Could you check a few things on this model? Use its own coordinates, in mm. A direction names the side the tool comes from. Give positions to 0.01 mm unless a question says otherwise; leave off trailing zeros. Order: outer loops, then holes, each group sorted by start corner. A loop starts at its lowest first (then second) coordinate and runs counter-clockwise, first axis right, second up. Notation, with made-up numbers: (-16, -6) - (34, -6) arc R19 cw to (34, 1) - close; hole circle Ø7 at (88.5, 12). An arc over 180 degrees is marked (long way). Put each result on its own line as item: value.
from build123d import *

# Parameters (mm, degrees)
EXTRUDE_THIN1_DEPTH             = 38.1
BOSS_EXTRUDE1_DEPTH             = 3.175
F_8_CLEARANCE_HOLE1_D           = 4.9149
FILLET1_R                       = 3.175
F_1_2_0_5_DIAMETER_HOLE1_D      = 12.7
F_9_64_0_14063_DIAMETER_HOLE1_D = 3.572002


with BuildPart() as part:
    # Sketch1 → Extrude-Thin1 (new body)
    with BuildSketch(Plane.XY):
        Polygon((-450.568590055, 3232.318777264), (-413.513639003, 3223.079940323), (-431.947583815, 3149.145425944), (-469.0030385, 3158.382242922), (-468.235104419, 3161.462973719), (-434.260212597, 3152.994048962), (-417.362429953, 3220.76735341), (-451.336692074, 3229.238088333), align=None)
    extrude(amount=-EXTRUDE_THIN1_DEPTH)

    # Sketch2 → Boss-Extrude1 (add)
    with BuildSketch(Plane(origin=(0, 0, -38.1), x_dir=(-1, 0, 0), z_dir=(0, 0, -1))):
        Polygon((413.513639003, 3223.079940323), (431.947583815, 3149.145425944), (469.0030385, 3158.382242922), (450.568590055, 3232.318777264), align=None)
    extrude(amount=-BOSS_EXTRUDE1_DEPTH)

    # #8 Clearance Hole1 (through all)
    with Locations(Plane.XY.offset(-34.925)):
        with Locations((-439.773757512, 3209.994133586), (-448.990981734, 3173.025866414)):
            Hole(F_8_CLEARANCE_HOLE1_D / 2)

    # Fillet1
    fillet1_edges = [part.edges().sort_by_distance(p)[0] for p in [
        (-413.513639003, 3223.079940323, -19.05),
        (-417.362429953, 3220.76735341, -17.4625),
        (-434.349561013, 3225.002720872, -34.925),
        (-451.247574539, 3157.228490409, -34.925),
        (-434.260212597, 3152.994048962, -17.4625),
        (-450.475311157, 3153.763834433, -38.1),
        (-431.947583815, 3149.145425944, -19.05),
        (-432.041114529, 3227.699358793, -38.1),
        (-422.730611409, 3186.112683133, -38.1),
    ]]
    fillet(fillet1_edges, radius=FILLET1_R - 0.0001)  # a hair under: the kernel refuses the full size

    # 1/2 (0.5) Diameter Hole1 (through all)
    with Locations(Plane(origin=(-1145.884443872, 285.70107988, 0), x_dir=(0, 0, -1), z_dir=(0.9702957262759976, -0.24192189559966307, 0))):
        with Locations((15.875, 2989.202688137)):
            Hole(F_1_2_0_5_DIAMETER_HOLE1_D / 2)

    # 9/64 (0.14063) Diameter Hole1 (through all)
    with Locations(Plane(origin=(-1145.884443872, 285.70107988, 0), x_dir=(0, 0, -1), z_dir=(0.9702957262759976, -0.24192189559966307, 0))):
        with Locations((15.875, 2979.677688137)):
            Hole(F_9_64_0_14063_DIAMETER_HOLE1_D / 2)


solid = part.part
1) We'd pull the mould along X, two halves only. Please class faces 4 (the flat face through (-420.735, 3194.117, -17.218)), 5 (the flat face through (-468.624, 3159.901, -18.783)), 6 (the cylindrical face through (-439.45, 3212.43, -36.53)): pulls with the +X half, pulls with the -X half, needs draft (parallel to the pull), parting line crosses it, or undercut.
Filled in:
face 4: pulls with the +X half
face 5: pulls with the -X half
face 6: undercut
2) I'm going to push flat-ended pins straight in: pin 1 (10 mm diameter, centred on x = -460.5, y = 3186, fed in from +Z) (3 decimals); pin 2 (5 mm diameter, centred on y = 3190.5, z = -5.5, fed in from -X); pin 3 (4 mm diameter, centred on y = 3160.5, z = -29.5, fed in from -X); pin 4 (4 mm diameter, centred on x = -439.77, y = 3209.99, fed in from +Z). Where does each tip first touch, or does it pass through?
Filled in:
pin 1: stops at z = -34.925
pin 2: stops at x = -425.53
pin 3: stops at x = -468.97
pin 4: passes through
3) Suppose I cut it at B-B, the plane z = -13. List the corners of the cut face in (x, y) for me.
Filled in:
outline: (-469, 3158.38) - (-435.03, 3149.91) arc R3.17 ccw to (-431.18, 3152.23) - (-424.1, 3180.62) - (-427.18, 3181.39) - (-433.49, 3156.07) arc R3.17 cw to (-437.34, 3153.76) - (-468.24, 3161.46) - close; (-451.34, 3229.24) - (-420.44, 3221.54) arc R3.17 cw to (-418.13, 3217.69) - (-424.44, 3192.37) - (-421.36, 3191.61) - (-414.28, 3220) arc R3.17 ccw to (-416.59, 3223.85) - (-450.57, 3232.32) - close
4) Suppose I cut it at A-A, the plane z = -24. List the corners of the cut face in (x, y) for me, and give its area (3 significant figures).
Filled in:
outline: (-469, 3158.38) - (-435.03, 3149.91) arc R3.17 ccw to (-431.18, 3152.23) - (-414.28, 3220) arc R3.17 ccw to (-416.59, 3223.85) - (-450.57, 3232.32) - (-451.34, 3229.24) - (-420.44, 3221.54) arc R3.17 cw to (-418.13, 3217.69) - (-433.49, 3156.07) arc R3.17 cw to (-437.34, 3153.76) - (-468.24, 3161.46) - close
area: 464 mm^2
5) If I drill on line 1 (Z direction, x = -448, y = 3177) (3 decimals); line 2 (Y direction, x = -442, z = -20); line 3 (X direction, y = 3202.5, z = -20.5), over which ranges is the centre line in solid material (lowest first)? Write a range as [from, to].
Filled in:
line 1: z = [-38.1, -34.925]
line 2: y = [3151.65, 3154.92], [3226.91, 3230.18]
line 3: x = [-421.92, -418.64]
6) Which directions (+Z, -Z, +X, -X, +Y, -Y) give clear straight access to the entire face, cutting with the end or side of a thin tool? Please do faces 1 (the cylindrical face through (-434.806, 3224.184, -33.97)), 2 (the cylindrical face through (-423.73, 3185.86, -37.15)), 3 (the cylindrical face through (-450.79, 3158.05, -33.97)).
Filled in:
face 1: +Z, -X
face 2: -Z, +X, -Y
face 3: +Z
